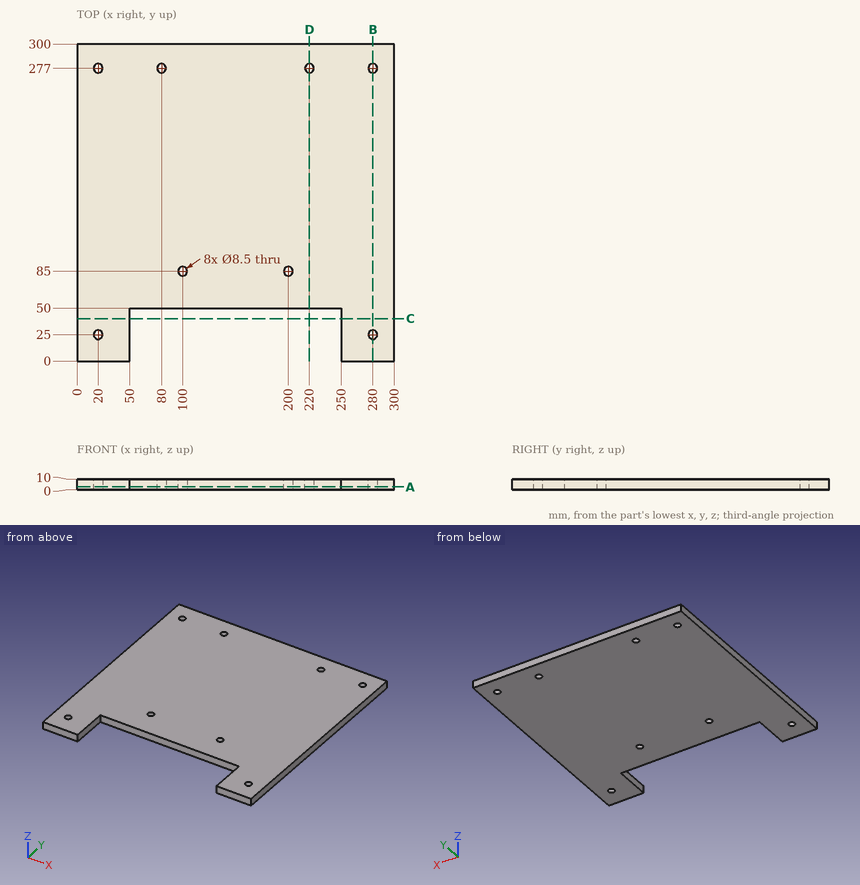
Geometry check sheet. Reference: drawing and pictorial views, mm from the part's lowest x, y, z. Coordinates: 2 decimals unless noted, no trailing zeros. Order: outer loops, then holes, each group sorted by start corner. A loop starts at its lowest first (then second) coordinate and runs counter-clockwise, first axis right, second up.
Item 1: Section check A-A, the plane z = 2.5. Give the number of separate pieces and of enclosed holes in the cut face, then the cut area to 3 significant figures.
Filled in:
separate pieces: 1
enclosed holes: 8
area: 79,500 mm2
Item 2: Depth check by flat-ended pin: pin 1 (5 mm diameter, centred on x = 158, z = 3.5, fed in from -Y). Enter the tip coordinate at first touch or a pass-through.
Filled in:
pin 1: stops at y = 50
Item 3: Section check D-D, the plane x = 220. Enter the section's corners in (y, z), then the cut area to 4 significant figures.
Filled in:
outline: (50, 0) - (272.75, 0) - (272.75, 10) - (50, 10) - close; (281.25, 0) - (300, 0) - (300, 10) - (281.25, 10) - close
area: 2,415 mm2
Item 4: Material ranges on L1, parallel to Y at x = 20, z = 3.25; L2, parallel to X at y = 277, z = 3.25; L3, parallel to X at y = 48, z = 6.5, recorded low to high.
Filled in:
L1: y = 0 to 20.75, 29.25 to 272.75, 281.25 to 300
L2: x = 0 to 15.75, 24.25 to 75.75, 84.25 to 215.75, 224.25 to 275.75, 284.25 to 300
L3: x = 0 to 50, 250 to 300
Item 5: Section check C-C, the plane y = 40. Enter the section's corners in (x, z), then the cut area to 3 significant figures.
Filled in:
outline: (0, 0) - (50, 0) - (50, 10) - (0, 10) - close; (250, 0) - (300, 0) - (300, 10) - (250, 10) - close
area: 1,000 mm2
Item 6: Section check B-B, the plane x = 280. Enter the section's corners in (y, z).
Filled in:
outline: (0, 0) - (20.75, 0) - (20.75, 10) - (0, 10) - close; (29.25, 0) - (272.75, 0) - (272.75, 10) - (29.25, 10) - close; (281.25, 0) - (300, 0) - (300, 10) - (281.25, 10) - close
